from build123d import *

# Parameters (mm, degrees)
SKETCH1_W            = 34.925
SKETCH1_H            = 60
BOSS_EXTRUDE1_DEPTH  = 1.5875
M4_CLEARANCE_HOLE1_D = 4.5
FILLET1_R            = 1.5875


with BuildPart() as part:
    # Sketch1 → Boss-Extrude1 (new body)
    with BuildSketch(Plane.XY):
        with Locations((-8.076586607, 43.274042014)):
            Rectangle(SKETCH1_W, SKETCH1_H)
    extrude(amount=-BOSS_EXTRUDE1_DEPTH)

    # M4 Clearance Hole1 (through all)
    with Locations(Plane(origin=(0, 0, -1.5875), x_dir=(-1, 0, 0), z_dir=(0, 0, -1))):
        with Locations((0.614086607, 63.594042014), (0.614086607, 22.954042014)):
            Hole(M4_CLEARANCE_HOLE1_D / 2)

    # Fillet1
    fillet1_edges = [part.edges().sort_by_distance(p)[0] for p in [
        (9.385913393, 13.274042014, -0.79375),
        (9.385913393, 73.274042014, -0.79375),
    ]]
    fillet(fillet1_edges, radius=FILLET1_R)


solid = part.part
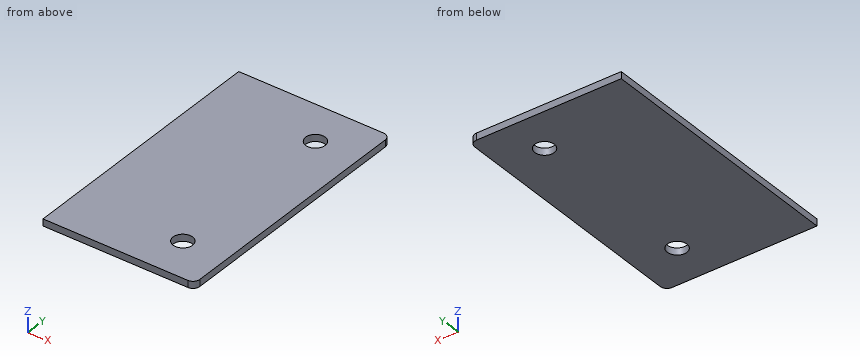
The listing builds one solid part. Answer for the finished solid, in the listing's coordinates (mm). Coordinates: 2 decimals unless noted, no trailing zeros. Write each loop counter-clockwise with the first axis right and the second up, starting at its lowest first coordinate (ties: lowest second). Pieces come first, ordered by that corner, then holes. Notation, with made-up numbers: (-39, 88) - (-20, 88) arc R14 ccw to (-20, 104) - close; hole circle Ø9 at (70, 22). An arc over 180 degrees is marked (long way). Answer as CSV lines item,"result".
1. Find section C-C (z = -0.4). Give the number of separate pieces and of enclosed holes in the cut face, plus the area to 3 significant figures.
Computed values:
separate pieces,"1"
enclosed holes,"2"
area,"2,060 mm²"
2. Find section B-B (y = 63). Give the vertices of the cut face in (x, z), plus the area to 3 significant figures.
Computed values:
outline,"(-25.54, -1.59) - (-2.78, -1.59) - (-2.78, 0) - (-25.54, 0) - close; (1.56, -1.59) - (9.39, -1.59) - (9.39, 0) - (1.56, 0) - close"
area,"48.6 mm²"
3. Straight lines are drawn through the part: line 1 (Y direction, x = 1, z = -1.4); line 2 (X direction, y = 23, z = -1.4); line 3 (X direction, y = 62.5, z = -0.95). For each, find the intervals that lie inside material, in ascending order. Write a range as [from, to].
Computed values:
line 1,"y = [13.27, 21.39], [24.52, 62.03], [65.16, 73.27]"
line 2,"x = [-25.54, -2.86], [1.64, 9.39]"
line 3,"x = [-25.54, -2.58], [1.35, 9.39]"
4. Find section A-A (x = -1.5). Give the vertices of the cut face in (y, z).
Computed values:
outline,"(13.27, -1.59) - (20.89, -1.59) - (20.89, 0) - (13.27, 0) - close; (25.02, -1.59) - (61.53, -1.59) - (61.53, 0) - (25.02, 0) - close; (65.66, -1.59) - (73.27, -1.59) - (73.27, 0) - (65.66, 0) - close"
